Read the model definition and answer for the solid it produces. Units are mm, in the model's axes. A direction names the side the tool comes from. Coordinates: 2 decimals unless noted, no trailing zeros. Loops run counter-clockwise (first coordinate to the right, second up) from the corner with the lowest first, then second, coordinate; pieces in that order, holes last.
from build123d import *

# Parameters (mm, degrees)
BOSS_EXTRUDE1_DEPTH  = 2
SKETCH1_3_W          = 3
SKETCH1_3_H          = 22
BOSS_EXTRUDE2_DEPTH  = 6.265
M3_CLEARANCE_HOLE1_D = 3.4
FILLET1_R            = 2
SKETCH6_R            = 1.625
CUT_EXTRUDE1_DEPTH   = 7.5
FILLET2_R            = 1
CHAMFER1_SIZE        = 0.5


with BuildPart() as part:
    # Sketch1 → Boss-Extrude1 (new body)
    with BuildSketch(Plane.XY):
        with BuildLine():
            Line((9.958333406, 3), (-4, 3))
            Line((-4, 3), (-4, -3))
            Line((-4, -3), (9.958333406, -3))
            ThreePointArc((9.958333406, -3), (10.44298868, -3.066896425), (10.891399918, -3.262582978))
            Line((10.891399918, -3.262582978), (11.642445292, -3.721657662))
            ThreePointArc((11.642445292, -3.721657662), (13.535102515, -4.547612803), (15.580738809, -4.829969693))
            Line((15.580738809, -4.829969693), (17.9, -4.829969693))
            Line((17.9, -4.829969693), (17.9, 4.829969693))
            Line((17.9, 4.829969693), (15.580738809, 4.829969693))
            ThreePointArc((15.580738809, 4.829969693), (13.535102515, 4.547612803), (11.642445292, 3.721657662))
            Line((11.642445292, 3.721657662), (10.891399918, 3.262582978))
            ThreePointArc((10.891399918, 3.262582978), (10.44298868, 3.066896425), (9.958333406, 3))
        make_face()
        Polygon((17.9, 11), (17.9, 4.829969693), (17.9, -4.829969693), (17.9, -11), (20.9, -11), (20.9, 11), align=None)
    extrude(amount=BOSS_EXTRUDE1_DEPTH)

    # Sketch1<3> → Boss-Extrude2 (add)
    with BuildSketch(Plane.XY):
        with Locations((19.4, 0)):
            Rectangle(SKETCH1_3_W, SKETCH1_3_H)
    extrude(amount=BOSS_EXTRUDE2_DEPTH)

    # M3 Clearance Hole1 (through all)
    with Locations(Plane.XY.offset(2)):
        with Locations((0, 0), (10, 0)):
            Hole(M3_CLEARANCE_HOLE1_D / 2)

    # Fillet1
    fillet1_edges = [part.edges().sort_by_distance(p)[0] for p in [
        (19.4, 11, 0),
        (19.4, -11, 0),
        (-4, -3, 1),
        (-4, 3, 1),
        (19.4, -11, 6.265),
        (19.4, 11, 6.265),
    ]]
    fillet(fillet1_edges, radius=FILLET1_R)

    # Sketch6 → Cut-Extrude1 (cut)
    with BuildSketch(Plane(origin=(20.9, 0, 0), x_dir=(0, 0, -1), z_dir=(1, 0, 0))):
        with Locations((-2.665, -8)):
            Circle(SKETCH6_R)
        with Locations((-2.665, 8)):
            Circle(SKETCH6_R)
    extrude(amount=-CUT_EXTRUDE1_DEPTH, mode=Mode.SUBTRACT)

    # Fillet2
    fillet2_edges = [part.edges().sort_by_distance(p)[0] for p in [
        (17.9, 0, 2),
    ]]
    fillet(fillet2_edges, radius=FILLET2_R)

    # Chamfer1
    chamfer1_edges = [part.edges().sort_by_distance(p)[0] for p in [
        (17.9, 4.829969693, 1),
        (17.9, -4.829969693, 1),
    ]]
    chamfer(chamfer1_edges, length=CHAMFER1_SIZE)


solid = part.part
Item 1: A cutting plane is placed at D-D on y = 4. Determine the outline of the cut face in (x, z) (3 decimals).
Numbers:
outline: (12.139, 0) - (20.9, 0) - (20.9, 6.265) - (17.9, 6.265) - (17.9, 3) arc R1 cw to (16.9, 2) - (12.139, 2) - close
Item 2: A cutting plane is placed at C-C on y = 0. Determine the outline of the cut face in (x, z) (3 decimals), then the cut area to 3 significant figures.
Numbers:
outline: (-4, 0) - (-1.7, 0) - (-1.7, 2) - (-4, 2) - close; (1.7, 0) - (8.3, 0) - (8.3, 2) - (1.7, 2) - close; (11.7, 0) - (20.9, 0) - (20.9, 6.265) - (17.9, 6.265) - (17.9, 3) arc R1 cw to (16.9, 2) - (11.7, 2) - close
area: 49.2 mm2
Item 3: Given pin 1 (5.5 mm diameter, centred on x = 0, y = 0, fed in from +Z); pin 2 (0.5 mm diameter, centred on x = 16.5, z = 1.5, fed in from +Y); pin 3 (2 mm diameter, centred on x = 5.5, z = 0.5, fed in from -Y); pin 4 (6 mm diameter, centred on x = 1.5, y = -4.5, fed in from -Z), each flat-ended and moving along its own axis, determine where each tip first touches the part or whether it passes through.
Numbers:
pin 1: stops at z = 2
pin 2: stops at y = 4.83
pin 3: stops at y = -3
pin 4: stops at z = 0
Item 4: Find the intervals of material crossed by line 1 along X through (y, z) = (1.5, 0.5); line 2 along Y through (x, z) = (18, 1.75); line 3 along X through (y, z) = (1.75, 4.5), in increasing order.
Numbers:
line 1: x = -3.94 to -0.8, 0.8 to 9.2, 10.8 to 20.9
line 2: y = -10.98 to -9.34, -6.66 to 6.66, 9.34 to 10.98
line 3: x = 17.9 to 20.9
Item 5: Which of the six approach directions +Z, -Z, +X, -X, +Y, -Y give full straight-line access (tool end or side, diameter ignored) to faces 4 (the face through (17, 4.83, 1)), 5 (the face through (6, 0, 2)), 6 (the face through (19.421, 10.43, 5.664))?
Numbers:
face 4: +Z, -Z, -X, +Y
face 5: +Z, -X, +Y, -Y
face 6: +Z, +X, -X, +Y
Item 6: A cutting plane is placed at B-B on y = 8. Determine the outline of the cut face in (x, z) (3 decimals), then the cut area to 4 significant figures.
Numbers:
outline: (17.9, 0) - (20.9, 0) - (20.9, 1.04) - (17.9, 1.04) - close; (17.9, 4.29) - (20.9, 4.29) - (20.9, 6.265) - (17.9, 6.265) - close
area: 9.045 mm2
Item 7: A cutting plane is placed at A-A on x = 0. Determine the outline of the cut face in (y, z), then the cut area to 3 significant figures.
Numbers:
outline: (-3, 0) - (-1.7, 0) - (-1.7, 2) - (-3, 2) - close; (1.7, 0) - (3, 0) - (3, 2) - (1.7, 2) - close
area: 5.20 mm2
Item 8: Determine the mould class of faces 1 (the face through (19, 0, 6.265)), 2 (the face through (19.42, -10.4, 0.57)), 3 (the face through (0.37, -1.66, 0.99)) for opening direction Y: released by +Y, released by -Y, zero draft, split by the parting line, or undercut.
Numbers:
face 1: zero draft
face 2: released by -Y
face 3: undercut
